The drawing under review shows one solid part. Ordinate dimensions are in mm from its lowest x, y, z. A direction names the side the tool comes from. Give positions to 0.01 mm unless a question says otherwise; leave off trailing zeros. Loops run counter-clockwise (first coordinate to the right, second up) from the corner with the lowest first, then second, coordinate; pieces in that order, holes last. Notation, with made-up numbers: (9, 67.5) - (55, 67.5) arc R32 cw to (55, 95.5) - close; hole circle Ø5 at (63, -7). An arc over 180 degrees is marked (long way). Answer as CSV lines item,"result".
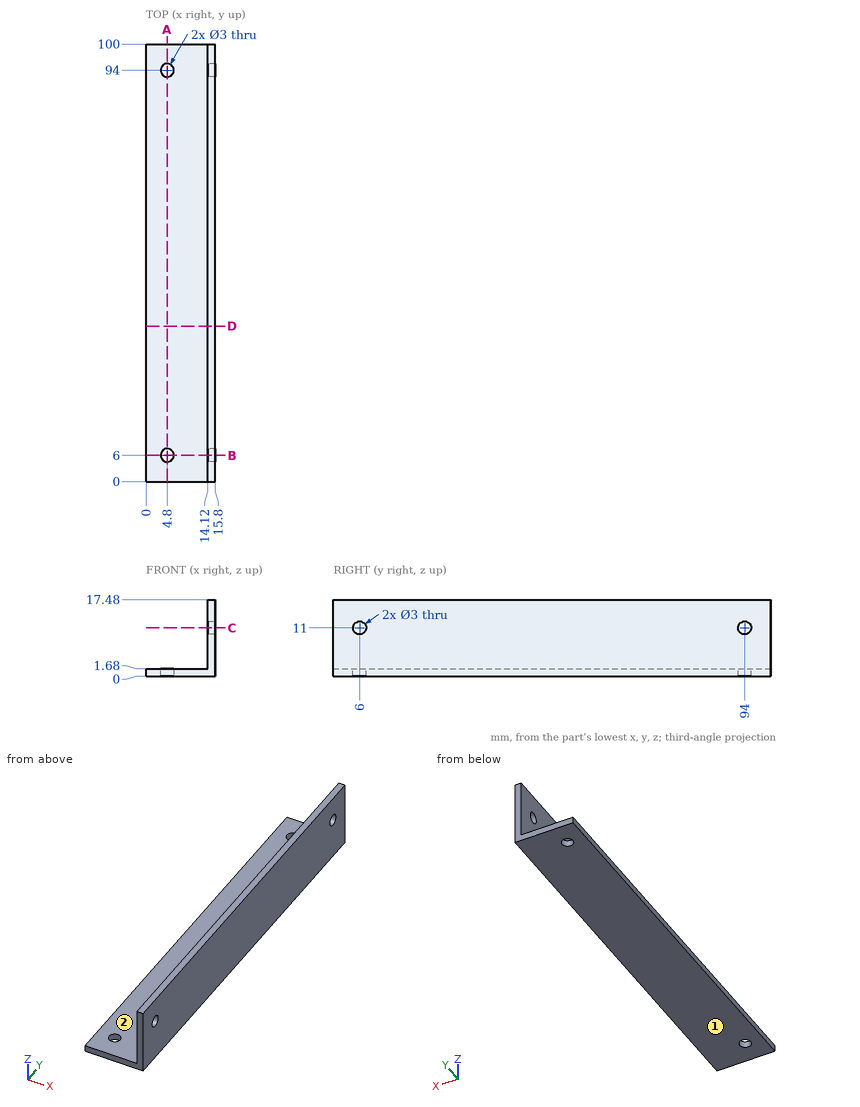
1) Insertion check: P1, Ø1, axis at x = 8.5, y = 80.5, coming from the -Z side; P2, Ø8, axis at y = 27.5, z = 6, coming from the -X side; P3, Ø3.5, axis at x = 4.8, y = 6, coming from the +Z side. Each pin has a flat end and moves straight along its axis. Give the tip position at first contact, or say it passes through.
From the geometry:
P1,"stops at z = 0"
P2,"stops at x = 14.12"
P3,"stops at z = 1.68"
2) Machinability: for the marked faces 1 and 2, which of the approach directions +Z, -Z, +X, -X, +Y, -Y give a long, thin tool a straight path to every point of the face, cutting with its end or side? Answer none if there is none.
From the geometry:
face 1,"-Z, +X, -X, +Y, -Y"
face 2,"+Z, -X, +Y, -Y"
3) Wall thickness on line 1 (Y direction, x = 14.7, z = 11); line 2 (Z direction, x = 7.75, y = 91.5); line 3 (X direction, y = 67, z = 10.75): over which ranges is each line inside the solid? List them lowest first. Write a range as from..to.
From the geometry:
line 1,"y = 0..4.5, 7.5..92.5, 95.5..100"
line 2,"z = 0..1.68"
line 3,"x = 14.12..15.8"
4) Consider section C-C on z = 11. Write out the cut boundary in (x, y), and give its area (3 significant figures).
From the geometry:
outline,"(14.12, 0) - (15.8, 0) - (15.8, 4.5) - (14.12, 4.5) - close; (14.12, 7.5) - (15.8, 7.5) - (15.8, 92.5) - (14.12, 92.5) - close; (14.12, 95.5) - (15.8, 95.5) - (15.8, 100) - (14.12, 100) - close"
area,"158 mm^2"
5) Consider section A-A on x = 4.8. Write out the cut boundary in (y, z).
From the geometry:
outline,"(0, 0) - (4.5, 0) - (4.5, 1.68) - (0, 1.68) - close; (7.5, 0) - (92.5, 0) - (92.5, 1.68) - (7.5, 1.68) - close; (95.5, 0) - (100, 0) - (100, 1.68) - (95.5, 1.68) - close"
6) Consider section D-D on y = 35.5. Write out the cut boundary in (x, z), and give its area (3 significant figures).
From the geometry:
outline,"(0, 0) - (15.8, 0) - (15.8, 17.48) - (14.12, 17.48) - (14.12, 1.68) - (0, 1.68) - close"
area,"53.1 mm^2"
7) Consider section B-B on y = 6. Write out the cut boundary in (x, z).
From the geometry:
outline,"(0, 0) - (3.3, 0) - (3.3, 1.68) - (0, 1.68) - close; (6.3, 0) - (15.8, 0) - (15.8, 9.5) - (14.12, 9.5) - (14.12, 1.68) - (6.3, 1.68) - close; (14.12, 12.5) - (15.8, 12.5) - (15.8, 17.48) - (14.12, 17.48) - close"
